Print and shaded views of the part. All mm, measured from the part's lowest x, y and z. Give positions to 0.01 mm unless a question says otherwise; leave off trailing zeros. Write each loop counter-clockwise with the first axis right and the second up, starting at its lowest first coordinate (ties: lowest second). Pieces come first, ordered by that corner, then holes. Notation, with made-up numbers: M 44,41.5 L 49,41.5 A19 ccw 49,54.5 Z; hole C 10,-32.75 d7. An arc over 180 degrees is marked long. One line per question, with ' | ' between items. Start each with the question number.
1. Cut at A-A, the plane x = 340. Write the cut outline in (y, z), then the cut area to 3 significant figures.
2. Cut at B-B, the plane z = 133.75. Write the cut outline in (x, y), then the cut area to 3 significant figures.
3. Flat gauge pin, fed straight in: pin 1 (6 mm diameter, centred on y = 6.5, z = 276, fed in from -X). Where does the tip first touch, or does it go through?
4. Wall check: L1, parallel to Z at x = 340, y = 7.5; L2, parallel to X at y = 3.25, z = 133.75; L3, parallel to X at y = 2, z = 267.5. Give the ranges that are in metal, low to high.
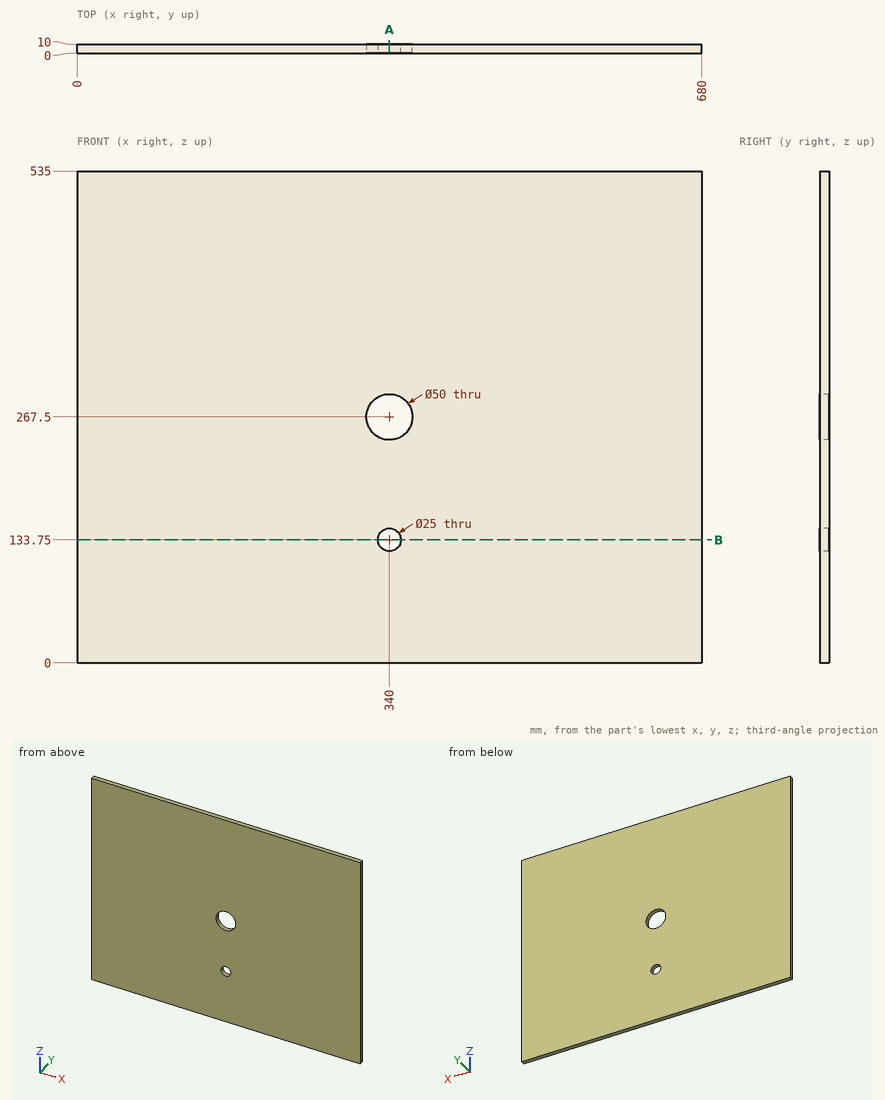
Here are the results:
1) outline: M 0,0 L 10,0 L 10,121.25 L 0,121.25 Z; M 0,146.25 L 10,146.25 L 10,242.5 L 0,242.5 Z; M 0,292.5 L 10,292.5 L 10,535 L 0,535 Z | area: 4,600 mm^2
2) outline: M 0,0 L 327.5,0 L 327.5,10 L 0,10 Z; M 352.5,0 L 680,0 L 680,10 L 352.5,10 Z | area: 6,550 mm^2
3) pin 1: x = 0
4) L1: 0 to 121.25, 146.25 to 242.5, 292.5 to 535 | L2: 0 to 327.5, 352.5 to 680 | L3: 0 to 315, 365 to 680
